Source: three-view drawing plus pictorial views. Frame: mm from the lowest corner of the part. A direction names the side the tool comes from. Give positions to 0.01 mm unless a question says otherwise; leave off trailing zeros. Order: outer loops, then holes, each group sorted by start corner. A loop starts at its lowest first (then second) coordinate and runs counter-clockwise, first axis right, second up. Notation, with made-up numbers: M -29,37 L 12,37 A13 cw 12,50 Z; hole C 30.5,81.25 d6. An arc over 180 degrees is marked long. Use CSV: the item, a comma, the result in double quotes. Start each with the question number.
1. Line query: line 1 along Z through (x, y) = (36.5, 8); line 2 along Z through (x, y) = (28, 29); line 3 along Y through (x, z) = (4.5, 21). Output: solid intervals per line, ascending. Write a range as [from, to].
2. Section query D-D, the plane y = 6.5. Return the cut outline in (x, z).
3. Section query C-C, the plane z = 29. Return the cut outline in (x, y), plus the area to 3 significant figures.
4. Pin query (flat end, axial travel): P1, Ø1.5, axis at x = 39.5, y = 14.5, coming from the +Z side; P2, Ø6, axis at x = 51, y = 17.5, coming from the +Z side; P3, Ø5, axis at x = 6, z = 33, coming from the -Y side. Return the tip coordinate at first contact, or that it passes through.
5. Section query B-B, the plane y = 35.5. Return the cut outline in (x, z).
6. Reachability of the marked faces 1, 2 and 3 from +Z, -Z, +X, -X, +Y, -Y: full face, straight path, thin tool, end or side. Return the list, or none.
7. Section query A-A, the plane x = 30. Return the cut outline in (y, z), plus the area to 3 significant figures.
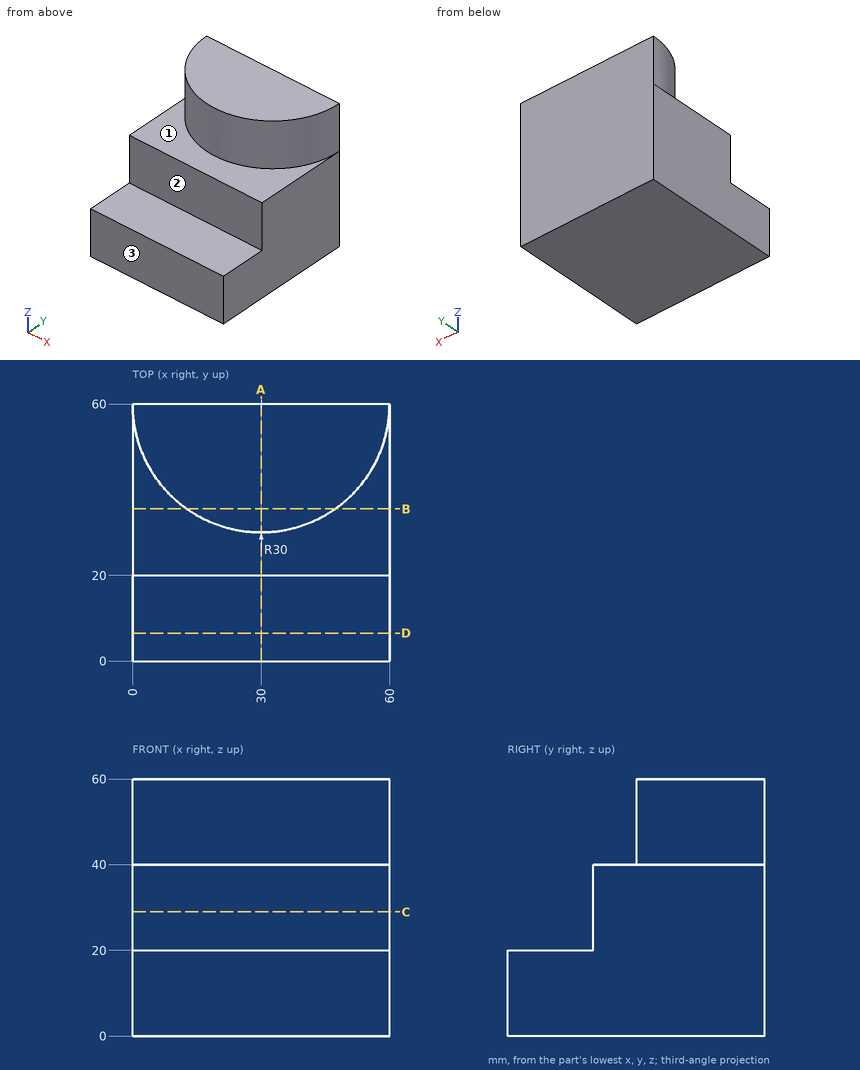
Result set:
1,line 1,"[0, 20]"
1,line 2,"[0, 40]"
1,line 3,"[20, 60]"
2,outline,"M 0,0 L 60,0 L 60,20 L 0,20 Z"
3,outline,"M 0,20 L 60,20 L 60,60 L 0,60 Z"
3,area,"2,400 mm2"
4,P1,"z = 20"
4,P2,"z = 40"
4,P3,"y = 20"
5,outline,"M 0,0 L 60,0 L 60,40 L 47.31,40 L 47.31,60 L 12.69,60 L 12.69,40 L 0,40 Z"
6,face 1,"+Z, -Y"
6,face 2,"+Z, +X, -X, -Y"
6,face 3,"+Z, -Z, +X, -X, -Y"
7,outline,"M 0,0 L 60,0 L 60,60 L 30,60 L 30,40 L 20,40 L 20,20 L 0,20 Z"
7,area,"2,600 mm2"
